Build history of the part. All positions in model axes, mm. A direction names the side the tool comes from. Give positions to 0.01 mm unless a question says otherwise; leave off trailing zeros. Order: outer loops, then holes, each group sorted by start corner. A loop starts at its lowest first (then second) coordinate and runs counter-clockwise, first axis right, second up. Notation, with made-up numbers: M 7.5,71 L 14.5,71 A25 cw 14.5,104 Z; hole C 19.5,-4.5 d3. An arc over 180 degrees is marked long. Answer as CSV lines item,"result".
from build123d import *

# Parameters (mm, degrees)
BOSS_EXTRUDE1_DEPTH             = 20
CUT_EXTRUDE2_DEPTH              = 25.109126902
CUT_EXTRUDE2_DEPTH_BACK         = 25.109126902
SKETCH2_R                       = 2.5
FILLET1_SIZE                    = 3
FILLET1_SIZE_2                  = 5
BOSS_EXTRUDE2_REACH             = 25.717
SKETCH3_W                       = 36
SKETCH3_H                       = 6
BOSS_EXTRUDE2_DIRECTION_2_REACH = 25.717


with BuildPart() as part:
    # Sketch1 → Boss-Extrude1 (new body)
    with BuildSketch(Plane.XY):
        Polygon((6.5, 2.5), (12.5, 2.5), (12.5, -2.5), (-12.5, -2.5), (-12.5, 2.5), align=None)
    extrude(amount=BOSS_EXTRUDE1_DEPTH)

    # Sketch2 → Cut-Extrude2 (cut, two sides: drawn at the far end of the back side and taken through both)
    with BuildSketch(Plane(origin=(0, 2.5, 0), x_dir=(1, 0, 0), z_dir=(0, 1, 0)).offset(-CUT_EXTRUDE2_DEPTH_BACK)):
        with Locations(Location((2, -10, 0), (0, 0, 270))):
            Circle(SKETCH2_R)
    extrude(amount=CUT_EXTRUDE2_DEPTH + CUT_EXTRUDE2_DEPTH_BACK, mode=Mode.SUBTRACT)

    # Fillet1
    # an asymmetric fillet: 5, 3 mm, written as the material it takes off along each edge
    with BuildSketch(Plane(origin=(12.5, 15, 20), x_dir=(0, 0, -1), z_dir=(0, -1, 0))) as fillet1_piece_1:
        with BuildLine():
            Bezier((FILLET1_SIZE, 0), (0, 0), (0, -FILLET1_SIZE_2), weights=[1, 0.707106781, 1])
            Line((0, -FILLET1_SIZE_2), (0, 0))
            Line((0, 0), (FILLET1_SIZE, 0))
        make_face()
    extrude(amount=30, mode=Mode.SUBTRACT)
    with BuildSketch(Plane(origin=(12.5, 15, 0), x_dir=(0, 0, 1), z_dir=(0, -1, 0))) as fillet1_piece_2:
        with BuildLine():
            Bezier((FILLET1_SIZE, 0), (0, 0), (0, FILLET1_SIZE_2), weights=[1, 0.707106781, 1])
            Line((0, FILLET1_SIZE_2), (0, 0))
            Line((0, 0), (FILLET1_SIZE, 0))
        make_face()
    extrude(amount=30, mode=Mode.SUBTRACT)

    # Boss-Extrude2: up to this face of the body (flat: up to its plane)
    boss_extrude2_end = Plane(part.part.faces().sort_by_distance((12.179843785, 2.5, 10))[0])
    # Sketch3 → Boss-Extrude2 (add, up to the picked face)
    with BuildSketch(Plane(origin=(0, 0, 0), x_dir=(1, 0, 0), z_dir=(0, 1, 0)), mode=Mode.PRIVATE) as boss_extrude2_sk1:
        with Locations((-30.5, -10)):
            Rectangle(SKETCH3_W, SKETCH3_H)
    boss_extrude2_tool1 = split(extrude(boss_extrude2_sk1.sketch, amount=BOSS_EXTRUDE2_REACH, mode=Mode.PRIVATE), bisect_by=boss_extrude2_end, keep=Keep.BOTH, mode=Mode.PRIVATE)
    add(boss_extrude2_tool1.solids().sort_by(Axis((-30.5, 0, 10), (0, 1, 0)))[0])

    # Boss-Extrude2 direction 2: up to this face of the body (flat: up to its plane)
    boss_extrude2_direction_2_end = Plane(part.part.faces().sort_by_distance((-2.5, -2.5, 0.320156215))[0])
    # Sketch3 → Boss-Extrude2 direction 2 (add, up to the picked face)
    with BuildSketch(Plane(origin=(0, 0, 0), x_dir=(1, 0, 0), z_dir=(0, 1, 0)), mode=Mode.PRIVATE) as boss_extrude2_direction_2_sk1:
        with Locations((-30.5, -10)):
            Rectangle(SKETCH3_W, SKETCH3_H)
    boss_extrude2_direction_2_tool1 = split(extrude(boss_extrude2_direction_2_sk1.sketch, amount=-BOSS_EXTRUDE2_DIRECTION_2_REACH, mode=Mode.PRIVATE), bisect_by=boss_extrude2_direction_2_end, keep=Keep.BOTH, mode=Mode.PRIVATE)
    add(boss_extrude2_direction_2_tool1.solids().sort_by(Axis((-30.5, 0, 10), (0, -1, 0)))[0])


solid = part.part
Item 1: 3-axis set-ups, long thin cutter, end or side, ignore diameter. For faces 1 (the flat face through (-48.5, 0, 10)), 2 (the flat face through (-31, 0, 7)), 3 (the flat face through (-12.5, 0, 16)): which of +Z, -Z, +X, -X, +Y, -Y reach the whole face in a straight line?
Geometry says:
face 1,"+Z, -Z, -X, +Y, -Y"
face 2,"-Z, -X, +Y, -Y"
face 3,"+Z, -X, +Y, -Y"
Item 2: Drop flat-ended pins along their axis: pin 1 (1.5 mm diameter, centred on x = -31.5, y = 0.5, fed in from -Z); pin 2 (8 mm diameter, centred on x = -18.5, z = 4.5, fed in from -Y). Give the stop position or say it passes through.
Geometry says:
pin 1,"stops at z = 7"
pin 2,"stops at y = -2.5"
Item 3: Probe line 1 along X through (y, z) = (-0.8, 10); line 2 along Z through (x, y) = (2, -0.3); line 3 along Z through (x, y) = (-38, 0.1). List the from-to ranges inside material, lowest first. Write a range as from..to.
Geometry says:
line 1,"x = -48.5..-0.5, 4.5..12.5"
line 2,"z = 0..7.5, 12.5..20"
line 3,"z = 7..13"
Item 4: Pull direction X, two halves, no side cores. Call faces 4 (the flat face through (-31, 0, 13)), 5 (the flat face through (12.5, 0, 10)), 6 (the cylindrical face through (-0.44, -0.04, 9.46)): released by +X, released by -X, zero draft, split by the parting line, or undercut.
Geometry says:
face 4,"zero draft"
face 5,"released by +X"
face 6,"undercut"
Item 5: Band-saw the part on A-A (z = 10). Give the cut face in (x, y), and give its area (3 significant figures).
Geometry says:
outline,"M -48.5,-2.5 L -0.5,-2.5 L -0.5,2.5 L -48.5,2.5 Z; M 4.5,-2.5 L 12.5,-2.5 L 12.5,2.5 L 4.5,2.5 Z"
area,"280 mm2"
Item 6: Band-saw the part on C-C (x = -42.5). Give the cut face in (y, z), and give its area (3 significant figures).
Geometry says:
outline,"M -2.5,7 L 2.5,7 L 2.5,13 L -2.5,13 Z"
area,"30.0 mm2"
Item 7: Band-saw the part on B-B (x = 2). Give the cut face in (y, z), and give its area (3 significant figures).
Geometry says:
outline,"M -2.5,0 L 2.5,0 L 2.5,7.5 L -2.5,7.5 Z; M -2.5,12.5 L 2.5,12.5 L 2.5,20 L -2.5,20 Z"
area,"75.0 mm2"
